The listing builds one solid part. Answer for the finished solid, in the listing's coordinates (mm). A direction names the side the tool comes from. Coordinates: 2 decimals unless noted, no trailing zeros. Loops run counter-clockwise (first coordinate to the right, second up) from the corner with the lowest first, then second, coordinate; pieces in that order, holes last. Notation, with made-up numbers: (4, 88.5) -> (18, 88.5) arc R17 cw to (18, 105.5) -> close; hole circle Ø1 at (18, 37). An arc over 180 degrees is marked (long way). Answer in a Markdown table with one row per item.
```python
from build123d import *

# Parameters (mm, degrees)
F0_W     = 70
F0_H     = 25
F0_R     = 1.75
F1_DEPTH = 3
F2_R     = 5
F2_R_2   = 1.75
F3_DEPTH = 20


with BuildPart() as f1:
    # F0 (on Top) → F1 (new body)
    with BuildSketch(Plane.XY):
        Rectangle(F0_W, F0_H)
        with Locations((-25, 0)):
            Circle(F0_R, mode=Mode.SUBTRACT)
        with BuildLine():
            ThreePointArc((26.75, 0), (25, -1.75), (23.25, 0))
            ThreePointArc((23.25, 0), (25, 1.75), (26.75, 0))
        make_face(mode=Mode.SUBTRACT)
    extrude(amount=F1_DEPTH)

    # F2 (on face) → F3 (join)
    with BuildSketch(Plane.XY.offset(3)):
        with Locations((-25, 0)):
            Circle(F2_R)
        with Locations((-25, 0)):
            Circle(F2_R_2, mode=Mode.SUBTRACT)
        with Locations((25, 0)):
            Circle(F2_R)
        with Locations((25, 0)):
            Circle(F2_R_2, mode=Mode.SUBTRACT)
    extrude(amount=-F3_DEPTH)


solid = f1.part
```
Item 1: A cutting plane is placed at C-C, the plane x = 28. Determine the outline of the cut face in (y, z).
Findings below:
| item | result |
|---|---|
| outline | (-12.5, 0) -> (-4, 0) -> (-4, -17) -> (4, -17) -> (4, 0) -> (12.5, 0) -> (12.5, 3) -> (-12.5, 3) -> close |
Item 2: A cutting plane is placed at B-B, the plane z = -8.75. Determine the outline of the cut face in (x, y), plus the area to 3 significant figures.
Findings below:
| item | result |
|---|---|
| outline | circle Ø10 at (-25, 0); circle Ø10 at (25, 0); hole circle Ø3.5 at (-25, 0); hole circle Ø3.5 at (25, 0) |
| area | 138 mm2 |
Item 3: Determine the mould class of faces 1 (the face through (-35, 0, 1)), 2 (the face through (0, 12.5, 1)), 3 (the face through (-30, 0, -8)) for opening direction X: +X half, -X half, draft (parallel to the pull), parting line (faces both ways), or undercut.
Findings below:
| item | result |
|---|---|
| face 1 | -X half |
| face 2 | draft |
| face 3 | undercut |
Item 4: A cutting plane is placed at D-D, the plane y = 10. Determine the outline of the cut face in (x, z), plus the area to 3 significant figures.
Findings below:
| item | result |
|---|---|
| outline | (-35, 0) -> (35, 0) -> (35, 3) -> (-35, 3) -> close |
| area | 210 mm2 |
Item 5: Find the intervals of material crossed by probe 1 along Y at (x, z) = (-25, 1.85); probe 2 along Y at (x, z) = (25, -11.25); probe 3 along Z at (x, y) = (9.5, 11), in increasing order.
Findings below:
| item | result |
|---|---|
| probe 1 | y = -12.5 to -1.75, 1.75 to 12.5 |
| probe 2 | y = -5 to -1.75, 1.75 to 5 |
| probe 3 | z = 0 to 3 |
Item 6: Flat-ended cylindrical pins translate along their axes: pin 1 Ø10 at (x, z) = (-22, -14.5) entering from +Y; pin 2 Ø10 at (x, z) = (-0.5, -7.5) entering from +Y; pin 3 Ø7.5 at (x, y) = (7, 1) entering from -Z; pin 4 Ø1 at (y, z) = (-2.5, -5) entering from +X. Find the tip coordinate at first contact, or state that the pin passes through.
Findings below:
| item | result |
|---|---|
| pin 1 | stops at y = 5 |
| pin 2 | passes through |
| pin 3 | stops at z = 0 |
| pin 4 | stops at x = 29.58 |
Item 7: A cutting plane is placed at A-A, the plane x = -25. Determine the outline of the cut face in (y, z), plus the area to 3 significant figures.
Findings below:
| item | result |
|---|---|
| outline | (-12.5, 0) -> (-5, 0) -> (-5, -17) -> (-1.75, -17) -> (-1.75, 3) -> (-12.5, 3) -> close; (1.75, -17) -> (5, -17) -> (5, 0) -> (12.5, 0) -> (12.5, 3) -> (1.75, 3) -> close |
| area | 175 mm2 |
Item 8: A tool of negligible diameter and unlimited length cuts with its end or side. For faces 4 (the face through (25, -2, -17)), 5 (the face through (20, 0, -8)), from which of +Z, -Z, +X, -X, +Y, -Y can it reach the whole face along a straight path? Write none if from no direction.
Findings below:
| item | result |
|---|---|
| face 4 | -Z, +X, -X, +Y, -Y |
| face 5 | -Z |
